Part print with two shaded views. Sizes in mm from the minimum x, y, z corner. A direction names the side the tool comes from. Coordinates: 2 decimals unless noted, no trailing zeros. Loops run counter-clockwise (first coordinate to the right, second up) from the corner with the lowest first, then second, coordinate; pieces in that order, holes last.
Item 1: Drill centre lines: line 1 along Y through (x, z) = (63, 5.75); line 2 along X through (y, z) = (19, 2); line 3 along X through (y, z) = (11, 9). Where is each one in solid material? Low to high.
Item 2: Cut at C-C (z = 3). List the corners of the cut face in (x, y), and give its area (3 significant figures).
Item 3: 3-axis set-ups, long thin cutter, end or side, ignore diameter. For the marked faces 1 and 2: which of +Z, -Z, +X, -X, +Y, -Y reach the whole face in a straight line?
Item 4: Cut at D-D (y = 19). List the corners of the cut face in (x, z), and give its area (3 significant figures).
Item 5: Cut at B-B (x = 63). List the corners of the cut face in (y, z).
Item 6: Cut at A-A (y = 3.5). List the corners of the cut face in (x, z).
Item 7: Flat gauge pin, fed straight in: pin 1 (2 mm diameter, centred on x = 28, z = 10.5, fed in from -Y). Where does the tip first touch, or does it go through?
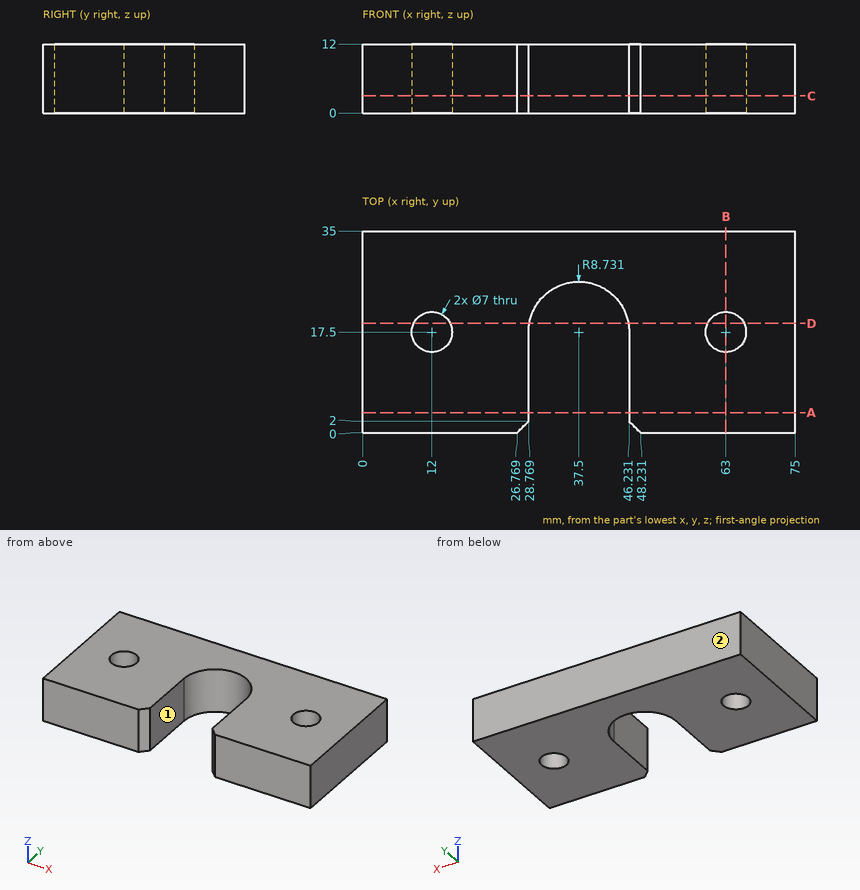
Filled sheet:
1. line 1: y = 0 to 14, 21 to 35
1. line 2: x = 0 to 8.84, 15.16 to 28.9, 46.1 to 59.84, 66.16 to 75
1. line 3: x = 0 to 28.77, 46.23 to 75
2. outline: (0, 0) - (26.77, 0) - (28.77, 2) - (28.77, 17.5) arc R8.73 cw to (46.23, 17.5) - (46.23, 2) - (48.23, 0) - (75, 0) - (75, 35) - (0, 35) - close; hole circle Ø7 at (12, 17.5); hole circle Ø7 at (63, 17.5)
2. area: 2,120 mm2
3. face 1: +Z, -Z, -Y
3. face 2: +Z, -Z, +X, -X, +Y
4. outline: (0, 0) - (8.84, 0) - (8.84, 12) - (0, 12) - close; (15.16, 0) - (28.9, 0) - (28.9, 12) - (15.16, 12) - close; (46.1, 0) - (59.84, 0) - (59.84, 12) - (46.1, 12) - close; (66.16, 0) - (75, 0) - (75, 12) - (66.16, 12) - close
4. area: 542 mm2
5. outline: (0, 0) - (14, 0) - (14, 12) - (0, 12) - close; (21, 0) - (35, 0) - (35, 12) - (21, 12) - close
6. outline: (0, 0) - (28.77, 0) - (28.77, 12) - (0, 12) - close; (46.23, 0) - (75, 0) - (75, 12) - (46.23, 12) - close
7. pin 1: stops at y = 0.23
